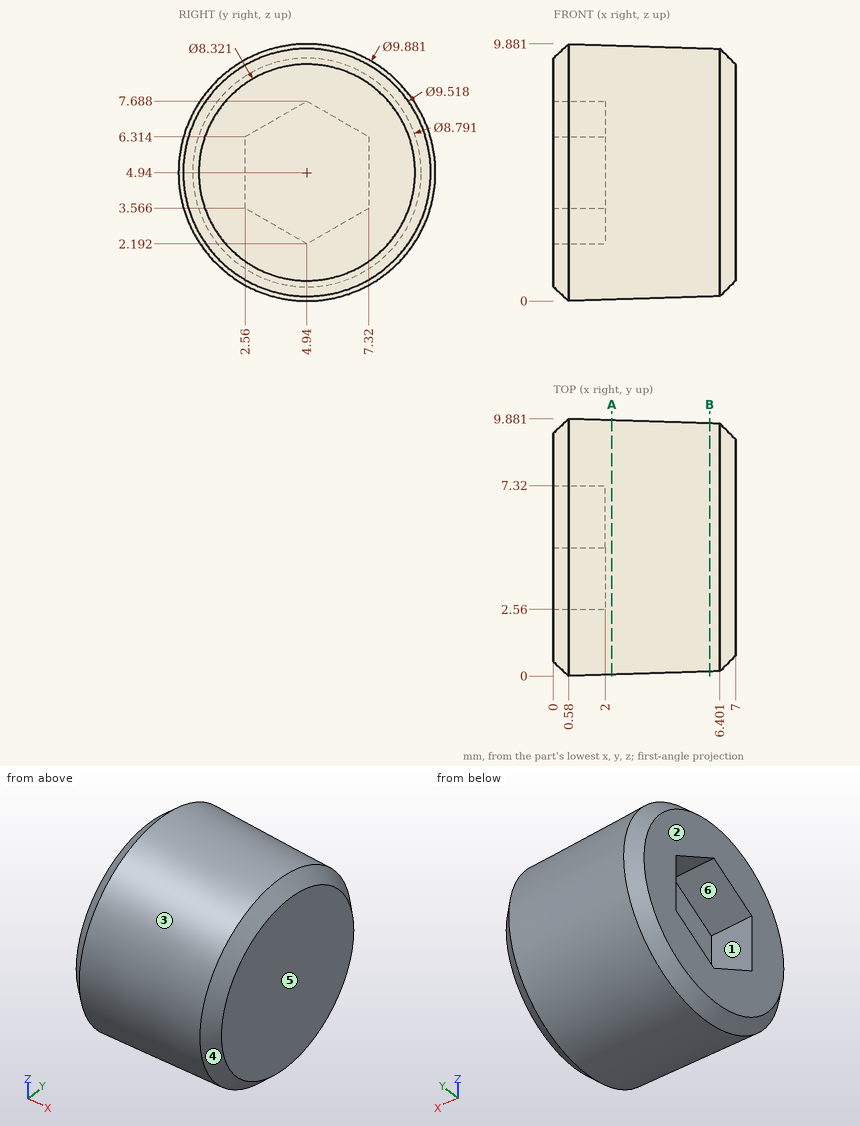
The figure shows three views and two pictorial views of one solid part (mm, origin at its lowest corner). Answer the questions. A direction names the side the tool comes from. Give positions to 0.01 mm unless a question says otherwise; leave off trailing zeros. Loops run counter-clockwise (first coordinate to the right, second up) from the corner with the lowest first, then second, coordinate; pieces in that order, holes last. Notation, with made-up numbers: (-40, 89) -> (-9, 89) arc R20 ccw to (-9, 96) -> close; hole circle Ø2 at (-20.75, 59). An arc over 180 degrees is marked (long way). Put each result on its own line as item: value. Start each with the question number.
Item 1: Each of these flat-tipped pins is pushed along its axis until it touches: P1, Ø3, axis at x = 5, z = 4.5, coming from the +Y side; P2, Ø1.4, axis at y = 4, z = 5.5, coming from the -X side; P3, Ø1.5, axis at x = 4.5, z = 4.5, coming from the -Y side. Where does it stop, or does it pass through?
Item 2: Find the intervals of material crossed by L1, parallel to Y at x = 1.75, z = 5; L2, parallel to Z at x = 0.5, y = 4.25 (1 decimal); L3, parallel to Y at x = 1.5, z = 5, in increasing order. Write a range as [from, to].
Item 3: The part is cut by section A-A (x = 2.25). Give the vertices of the cut face in (y, z).
Item 4: The mould has two halves that part along Z. Classify the marked faces 4, 5 and 6: released by +Z, released by -Z, zero draft, split by the parting line, or undercut.
Item 5: Which of the six approach directions +Z, -Z, +X, -X, +Y, -Y give full straight-line access (tool end or side, diameter ignored) to the marked faces 1, 2 and 3?
Item 6: The part is cut by section B-B (x = 6). Give the vertices of the cut face in (y, z).
Answers below:
1. P1: y = 9.79
1. P2: x = 2
1. P3: y = 0.1
2. L1: [0.04, 2.56], [7.32, 9.84]
2. L2: [0.1, 2.6], [7.3, 9.8]
2. L3: [0.03, 2.56], [7.32, 9.85]
3. outline: circle Ø9.78 at (4.94, 4.94)
4. face 4: split by the parting line
4. face 5: zero draft
4. face 6: undercut
5. face 1: -X
5. face 2: +Z, -Z, -X, +Y, -Y
5. face 3: +X
6. outline: circle Ø9.54 at (4.94, 4.94)
